Input: part model. Units: mm. Frame: model coordinates. Face numbers are marked on the shaded views. Coordinates: 2 decimals unless noted, no trailing zeros. Order: outer loops, then holes, each group sorted by start corner. A loop starts at its lowest first (then second) coordinate and runs counter-clockwise, first axis right, second up. Notation, with made-up numbers: (60, -10) - (102, -10) arc R9 ccw to (102, -5) - close; hole circle Ø5 at (80, -27). An arc over 180 degrees is marked (long way). Use a Markdown table: item, result. Add a question column.
from build123d import *

# Parameters (mm, degrees)
F1_DEPTH = 368.3
F2_W     = 452.085844
F2_H     = 300.708675
F2_W_2   = 450.040182
F2_H_2   = 272.069744
F3_DEPTH = 381
F4_W     = 46.388466
F4_H     = 111.5514
F4_W_2   = 66.730906
F4_H_2   = 130.886974
F5_DEPTH = 12.7


with BuildPart() as f1:
    # F0 (on Top) → F1 (new body)
    with BuildSketch(Plane.XY):
        with BuildLine():
            Line((458.216, -9.525), (533.4, -9.525))
            Line((533.4, -9.525), (533.4, 9.525))
            Line((533.4, 9.525), (-533.4, 9.525))
            Line((-533.4, 9.525), (-533.4, -9.525))
            Line((-533.4, -9.525), (-509.016, -9.525))
            ThreePointArc((-509.016, -9.525), (-508.29758, -9.22742), (-508, -8.509))
            ThreePointArc((-508, -8.509), (-507.70242, -9.22742), (-506.984, -9.525))
            Line((-506.984, -9.525), (-458.216, -9.525))
            ThreePointArc((-458.216, -9.525), (-457.49758, -9.22742), (-457.2, -8.509))
            ThreePointArc((-457.2, -8.509), (-456.90242, -9.22742), (-456.184, -9.525))
            Line((-456.184, -9.525), (-407.416, -9.525))
            ThreePointArc((-407.416, -9.525), (-406.69758, -9.22742), (-406.4, -8.509))
            ThreePointArc((-406.4, -8.509), (-406.10242, -9.22742), (-405.384, -9.525))
            Line((-405.384, -9.525), (-356.616, -9.525))
            ThreePointArc((-356.616, -9.525), (-355.89758, -9.22742), (-355.6, -8.509))
            ThreePointArc((-355.6, -8.509), (-355.30242, -9.22742), (-354.584, -9.525))
            Line((-354.584, -9.525), (-305.816, -9.525))
            ThreePointArc((-305.816, -9.525), (-305.09758, -9.22742), (-304.8, -8.509))
            ThreePointArc((-304.8, -8.509), (-304.50242, -9.22742), (-303.784, -9.525))
            Line((-303.784, -9.525), (-255.016, -9.525))
            ThreePointArc((-255.016, -9.525), (-254.29758, -9.22742), (-254, -8.509))
            ThreePointArc((-254, -8.509), (-253.70242, -9.22742), (-252.984, -9.525))
            Line((-252.984, -9.525), (-204.216, -9.525))
            ThreePointArc((-204.216, -9.525), (-203.49758, -9.22742), (-203.2, -8.509))
            ThreePointArc((-203.2, -8.509), (-202.90242, -9.22742), (-202.184, -9.525))
            Line((-202.184, -9.525), (-153.416, -9.525))
            ThreePointArc((-153.416, -9.525), (-152.69758, -9.22742), (-152.4, -8.509))
            ThreePointArc((-152.4, -8.509), (-152.10242, -9.22742), (-151.384, -9.525))
            Line((-151.384, -9.525), (-102.616, -9.525))
            ThreePointArc((-102.616, -9.525), (-101.89758, -9.22742), (-101.6, -8.509))
            ThreePointArc((-101.6, -8.509), (-101.30242, -9.22742), (-100.584, -9.525))
            Line((-100.584, -9.525), (-51.816, -9.525))
            ThreePointArc((-51.816, -9.525), (-51.09758, -9.22742), (-50.8, -8.509))
            ThreePointArc((-50.8, -8.509), (-50.50242, -9.22742), (-49.784, -9.525))
            Line((-49.784, -9.525), (-1.016, -9.525))
            ThreePointArc((-1.016, -9.525), (-0.29758, -9.22742), (0, -8.509))
            ThreePointArc((0, -8.509), (0.29758, -9.22742), (1.016, -9.525))
            Line((1.016, -9.525), (49.784, -9.525))
            ThreePointArc((49.784, -9.525), (50.50242, -9.22742), (50.8, -8.509))
            ThreePointArc((50.8, -8.509), (51.09758, -9.22742), (51.816, -9.525))
            Line((51.816, -9.525), (100.584, -9.525))
            ThreePointArc((100.584, -9.525), (101.30242, -9.22742), (101.6, -8.509))
            ThreePointArc((101.6, -8.509), (101.89758, -9.22742), (102.616, -9.525))
            Line((102.616, -9.525), (151.384, -9.525))
            ThreePointArc((151.384, -9.525), (152.10242, -9.22742), (152.4, -8.509))
            ThreePointArc((152.4, -8.509), (152.69758, -9.22742), (153.416, -9.525))
            Line((153.416, -9.525), (202.184, -9.525))
            ThreePointArc((202.184, -9.525), (202.90242, -9.22742), (203.2, -8.509))
            ThreePointArc((203.2, -8.509), (203.49758, -9.22742), (204.216, -9.525))
            Line((204.216, -9.525), (252.984, -9.525))
            ThreePointArc((252.984, -9.525), (253.70242, -9.22742), (254, -8.509))
            ThreePointArc((254, -8.509), (254.29758, -9.22742), (255.016, -9.525))
            Line((255.016, -9.525), (303.784, -9.525))
            ThreePointArc((303.784, -9.525), (304.50242, -9.22742), (304.8, -8.509))
            ThreePointArc((304.8, -8.509), (305.09758, -9.22742), (305.816, -9.525))
            Line((305.816, -9.525), (354.584, -9.525))
            ThreePointArc((354.584, -9.525), (355.30242, -9.22742), (355.6, -8.509))
            ThreePointArc((355.6, -8.509), (355.89758, -9.22742), (356.616, -9.525))
            Line((356.616, -9.525), (405.384, -9.525))
            ThreePointArc((405.384, -9.525), (406.10242, -9.22742), (406.4, -8.509))
            ThreePointArc((406.4, -8.509), (406.69758, -9.22742), (407.416, -9.525))
            Line((407.416, -9.525), (456.184, -9.525))
            ThreePointArc((456.184, -9.525), (456.90242, -9.22742), (457.2, -8.509))
            ThreePointArc((457.2, -8.509), (457.49758, -9.22742), (458.216, -9.525))
        make_face()
        with BuildLine():
            ThreePointArc((-508, -8.509), (-508.29758, -9.22742), (-509.016, -9.525))
            Line((-509.016, -9.525), (-506.984, -9.525))
            ThreePointArc((-506.984, -9.525), (-507.70242, -9.22742), (-508, -8.509))
        make_face()
    extrude(amount=F1_DEPTH)

    # F2 (on Top) → F3 (cut)
    with BuildSketch(Plane.XY):
        with Locations((-378.442922, -15.51013)):
            Rectangle(F2_W, F2_H)
        with Locations((377.420091, 0.854973)):
            Rectangle(F2_W_2, F2_H_2)
    extrude(amount=F3_DEPTH, mode=Mode.SUBTRACT)

    # F4 (on Front) → F5 (cut, symmetric)
    with BuildSketch(Plane.XZ):
        with Locations((-155.528233, 373.2757)):
            Rectangle(F4_W, F4_H)
        with Locations((165.699453, 382.943487)):
            Rectangle(F4_W_2, F4_H_2)
    extrude(amount=F5_DEPTH, both=True, mode=Mode.SUBTRACT)


solid = f1.part
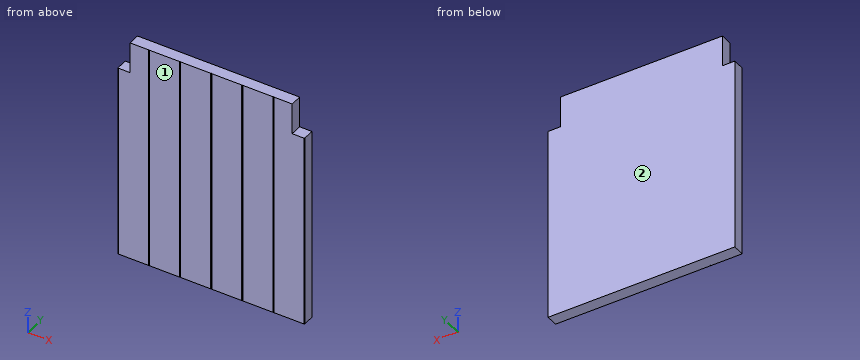
1) Contact query for flat-ended pins moving along their axis: P1, Ø9.5, axis at x = -146.5, y = 3, coming from the +Z side; P2, Ø5.5, axis at y = -3, z = 343.5, coming from the -X side. Output: stop coordinate, or through.
2) Pull-direction query (Y, two-part tool) for the marked faces 1 and 2; classes: pulls with the +Y half, pulls with the -Y half, needs draft (parallel to the pull), parting line crosses it, or undercut.
3) Material intervals for L1, parallel to Z at x = -136, y = 3.5; L2, parallel to X at y = 4.5, z = 335, sorted ascending.
4) Cut plane A-A (y = 2.25). Return the cut outline in (x, z).
Computed:
| question | item | result |
|---|---|---|
| 1 | P1 | stops at z = 317.5 |
| 1 | P2 | stops at x = -132.33 |
| 2 | face 1 | pulls with the -Y half |
| 2 | face 2 | pulls with the +Y half |
| 3 | L1 | z = 0 to 317.5 |
| 3 | L2 | x = -132.33 to 132.33 |
| 4 | outline | (-152.4, 0) - (152.4, 0) - (152.4, 317.5) - (132.33, 317.5) - (132.33, 368.3) - (-132.33, 368.3) - (-132.33, 317.5) - (-152.4, 317.5) - close |
